The figure shows three views and two pictorial views of one solid part (mm, origin at its lowest corner). Answer the questions. A direction names the side the tool comes from. Give positions to 0.01 mm unless a question says otherwise; leave off trailing zeros. Write each loop counter-clockwise with the first axis right and the second up, starting at its lowest first coordinate (ties: lowest second). Pieces come first, ordered by that corner, then holes. Notation, with made-up numbers: (-28, 63) - (6, 63) arc R12 cw to (6, 78) - close; hole circle Ø10 at (-3.75, -28). An arc over 180 degrees is marked (long way). One line per question, with ' | ' between items. Start each with the question number.
1. Find the intervals of material crossed by L1, parallel to Y at x = 80.5, z = 80; L2, parallel to Z at x = 215, y = 87, in increasing order. Write a range as from..to.
2. A cutting plane is placed at C-C (z = 234). Determine the outline of the cut face in (x, y).
3. A cutting plane is placed at B-B (y = 63.5). Determine the outline of the cut face in (x, z), then the cut area to 3 significant figures.
4. The mould has two halves that part along Y. Classify the marked faces 6, 7 and 8: +Y half, -Y half, draft (parallel to the pull), parting line (faces both ways), or undercut.
5. Given P1, Ø10, axis at x = 175.5, y = 216.5, coming from the +Z side, flat-ended and moving along its own axis, determine where the tip first touches the part or whether it passes through.
6. A cutting plane is placed at D-D (x = 106.5). Determine the outline of the cut face in (y, z), then the cut area to 3 significant figures.
7. For the marked faces 1, 2, 3, 4 and 5, determine the directions among +Z, -Z, +X, -X, +Y, -Y from which every point of the face is accessible in a straight line to the end or side of a thin tool.
8. A cutting plane is placed at A-A (x = 203). Determine the outline of the cut face in (y, z).
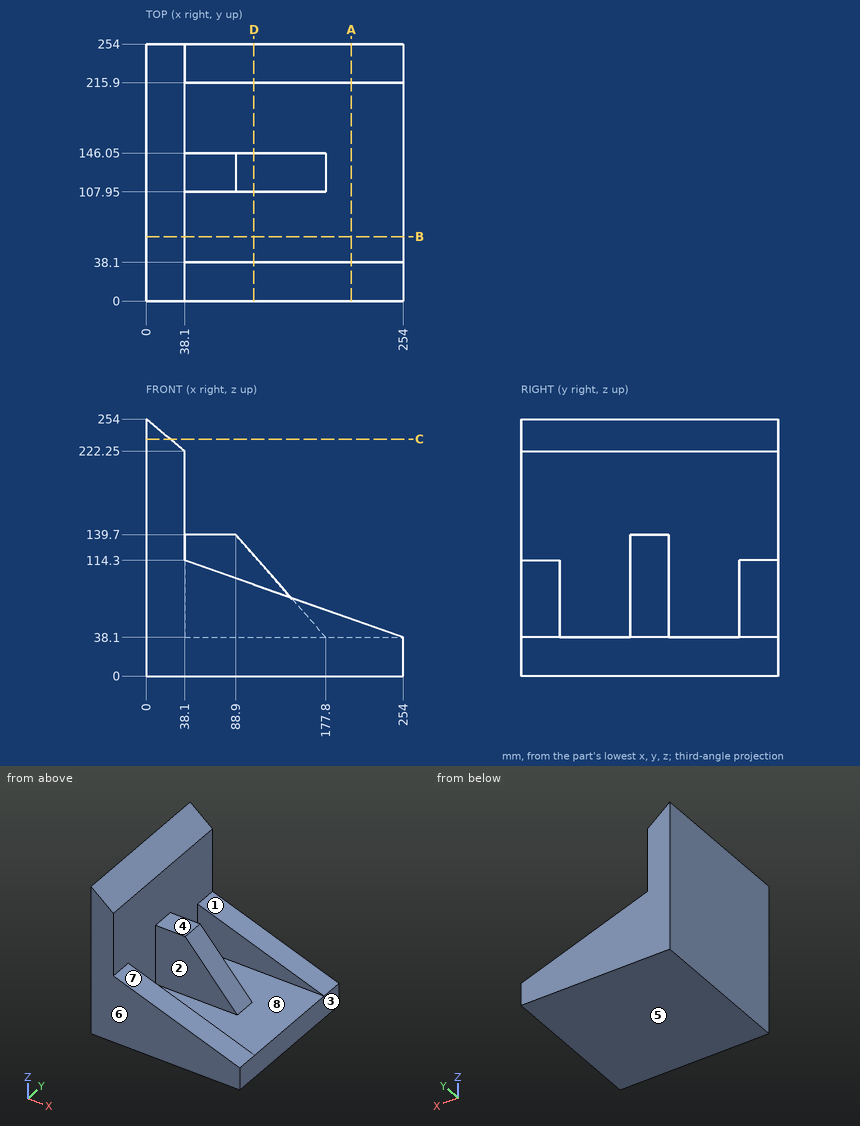
Determined:
1) L1: 0..38.1, 107.95..146.05, 215.9..254 | L2: 0..38.1
2) outline: (0, 0) - (24, 0) - (24, 254) - (0, 254) - close
3) outline: (0, 0) - (254, 0) - (254, 38.1) - (38.1, 38.1) - (38.1, 222.25) - (0, 254) - close | area: 17,300 mm2
4) face 6: -Y half | face 7: draft | face 8: undercut
5) P1: z = 67.57
6) outline: (0, 0) - (254, 0) - (254, 90.16) - (215.9, 90.16) - (215.9, 38.1) - (146.05, 38.1) - (146.05, 119.59) - (107.95, 119.59) - (107.95, 38.1) - (38.1, 38.1) - (38.1, 90.16) - (0, 90.16) - close | area: 16,700 mm2
7) face 1: +Z, +X, +Y | face 2: +Z, +X | face 3: +Z, -Z, +X, +Y, -Y | face 4: +Z, +X, +Y, -Y | face 5: -Z, +X, -X, +Y, -Y
8) outline: (0, 0) - (254, 0) - (254, 56.1) - (215.9, 56.1) - (215.9, 38.1) - (38.1, 38.1) - (38.1, 56.1) - (0, 56.1) - close
